```python
from build123d import *

# Parameters (mm, degrees)
F0_W     = 76.2
F0_H     = 50.8
F0_W_2   = 69.85
F0_H_2   = 44.45
F2_DEPTH = 193.04
F3_R     = 3.175
F4_R     = 3
F5_DEPTH = 25.4
F7_DEPTH = 25.4


# Not quite as in the source:
# - a variable given as a bare number and used for a length is read in inches; the dataset says mm whatever the document's units were


with BuildPart() as f2:
    # F0 (on Front) → F2 (new body)
    with BuildSketch(Plane.XZ):
        Rectangle(F0_W, F0_H)
        Rectangle(F0_W_2, F0_H_2, mode=Mode.SUBTRACT)
    extrude(amount=F2_DEPTH)

    # F3
    f3_edges = [f2.edges().sort_by_distance(p)[0] for p in [
        (-38.1, -96.52, -25.4),
        (-38.1, -96.52, 25.4),
        (38.1, -96.52, -25.4),
        (38.1, -96.52, 25.4),
        (-34.925, -96.52, -22.225),
        (-34.925, -96.52, 22.225),
        (34.925, -96.52, 22.225),
        (34.925, -96.52, -22.225),
    ]]
    fillet(f3_edges, radius=F3_R)

    # F4 (on face) → F5 (cut)
    with BuildSketch(Plane(origin=(0, 0, -25.4), x_dir=(1, 0, 0), z_dir=(0, 0, -1))):
        with Locations((-12.7, 58.42)):
            Circle(F4_R)
        with Locations((12.7, 58.42)):
            Circle(F4_R)
        with Locations((12.7, 134.62)):
            Circle(F4_R)
        with Locations((-12.7, 134.62)):
            Circle(F4_R)
    extrude(amount=-F5_DEPTH, mode=Mode.SUBTRACT)

    # F6 (on face) → F7 (cut)
    with BuildSketch(Plane.XY.offset(25.4)):
        Polygon((34.925, -33.02), (0, -33.02), (-34.925, -33.02), (-34.925, -160.02), (34.925, -160.02), align=None)
    extrude(amount=-F7_DEPTH, mode=Mode.SUBTRACT)


solid = f2.part
```
Input: part model. Units: mm. Frame: model coordinates. A direction names the side the tool comes from. Round coordinates to 2 decimals unless told otherwise and drop trailing zeros. Loops run counter-clockwise (first coordinate to the right, second up) from the corner with the lowest first, then second, coordinate; pieces in that order, holes last. Notation, with made-up numbers: (-25.75, -35) - (20.25, -35) arc R22 cw to (20.25, -10) - close; hole circle Ø8 at (31.5, -13). An arc over 180 degrees is marked (long way). One line per item, written item: value. Start each with the question number.
(1) Section C-C, the plane y = -58.42. Return loops of the section in (x, z) (3 decimals).
(2) Section A-A, the plane x = -12.7. Return loops of the section in (y, z) (3 decimals), plus the area to 3 significant figures.
(3) Contact query for flat-ended pins moving along their axis: P1, Ø5.5, axis at x = -12.7, y = -58.42, coming from the -Z side; P2, Ø3, axis at x = -22.5, y = -96.5, coming from the +Z side (3 decimals). Output: stop coordinate, or through.
(4) Section B-B, the plane z = -3. Return loops of the section in (x, y) (3 decimals).
(5) Ray query, line 1 (Y direction, x = -12.7, z = -23.7); line 2 (X direction, y = -10.5, z = -9) (3 decimals); line 3 (Y direction, x = -12, z = -23). Return the intervals inside material, ascending. Write a range as [from, to].
(6) Section D-D, the plane x = -3. Return loops of the section in (y, z) (3 decimals).
(7) Draft query along Y for faces 3 (the flat face through (-3, -193.04, -22.5)), 4 (the flat face through (0, -33.02, 24)), 5 (the flat face through (0, -16, 22.225)), 6 (the flat face through (0, -160.02, 24)). Return one class per face: +Y half, -Y half, draft (parallel to the pull), parting line (faces both ways), or undercut.
(8) Access query for faces 1 (the cylindrical face through (14.31, -137.15, -23.83)), 2 (the flat face through (0, -95, -22.225)). Directions: +Z, -Z, +X, -X, +Y, -Y. A direction counts if a zero-diameter tool reaches every point of the face in a straight line with its end or side. Return the directions, or none.
Results below:
1. outline: (-38.1, -22.225) arc R3.175 ccw to (-34.925, -25.4) - (-15.7, -25.4) - (-15.7, -22.225) - (-31.75, -22.225) arc R3.175 cw to (-34.925, -19.05) - (-34.925, 25.4) arc R3.175 ccw to (-38.1, 22.225) - close; (-9.7, -25.4) - (9.7, -25.4) - (9.7, -22.225) - (-9.7, -22.225) - close; (15.7, -25.4) - (34.925, -25.4) arc R3.175 ccw to (38.1, -22.225) - (38.1, 22.225) arc R3.175 ccw to (34.925, 25.4) - (34.925, -19.05) arc R3.175 cw to (31.75, -22.225) - (15.7, -22.225) - close
2. outline: (-193.04, -25.4) - (-137.62, -25.4) - (-137.62, -22.225) - (-193.04, -22.225) - close; (-193.04, 22.225) - (-160.02, 22.225) - (-160.02, 25.4) - (-193.04, 25.4) - close; (-131.62, -25.4) - (-61.42, -25.4) - (-61.42, -22.225) - (-131.62, -22.225) - close; (-55.42, -25.4) - (0, -25.4) - (0, -22.225) - (-55.42, -22.225) - close; (-33.02, 22.225) - (0, 22.225) - (0, 25.4) - (-33.02, 25.4) - close
2. area: 784 mm^2
3. P1: through
3. P2: z = -22.225
4. outline: (-38.1, -193.04) - (-34.925, -193.04) - (-34.925, 0) - (-38.1, 0) - close; (34.925, -193.04) - (38.1, -193.04) - (38.1, 0) - (34.925, 0) - close
5. line 1: [-193.04, -137.62], [-131.62, -61.42], [-55.42, 0]
5. line 2: [-38.1, -34.925], [34.925, 38.1]
5. line 3: [-193.04, -137.54], [-131.7, -61.34], [-55.5, 0]
6. outline: (-193.04, -25.4) - (0, -25.4) - (0, -22.225) - (-193.04, -22.225) - close; (-193.04, 22.225) - (-160.02, 22.225) - (-160.02, 25.4) - (-193.04, 25.4) - close; (-33.02, 22.225) - (0, 22.225) - (0, 25.4) - (-33.02, 25.4) - close
7. face 3: -Y half
7. face 4: undercut
7. face 5: draft
7. face 6: undercut
8. face 1: +Z, -Z
8. face 2: +Y, -Y
